from build123d import *

# Parameters (mm, degrees)
SKETCH1_R           = 25
BOSS_EXTRUDE1_DEPTH = 100
SKETCH2_R           = 35
BOSS_EXTRUDE2_DEPTH = 10


with BuildPart() as part:
    # Sketch1 → Boss-Extrude1 (new body)
    with BuildSketch(Plane.XY):
        Circle(SKETCH1_R)
    extrude(amount=BOSS_EXTRUDE1_DEPTH)

    # Sketch2 → Boss-Extrude2 (add)
    with BuildSketch(Plane.XY.offset(100)):
        Circle(SKETCH2_R)
    boss_extrude2 = extrude(amount=BOSS_EXTRUDE2_DEPTH)

    # Mirror1: Boss-Extrude2 across plane
    add(boss_extrude2.mirror(Plane(origin=(0, 0, 50), x_dir=(1, 0, 0), z_dir=(0, 0, -1))))


solid = part.part
Verification items for the finished model (mm, model axes). A direction names the side the tool comes from. Give positions to 0.01 mm unless a question says otherwise; leave off trailing zeros. Loops run counter-clockwise (first coordinate to the right, second up) from the corner with the lowest first, then second, coordinate; pieces in that order, holes last.
1) Sectioned sample at A-A, the plane y = 0. Enter the section's corners in (x, z), then the cut area to 3 significant figures.
2) Sectioned sample at D-D, the plane z = 59.5. Enter the section's corners in (x, y).
3) Draft check along Z on faces 1 (the flat face through (-24, 8, 100)), 2 (the flat face through (0, 0, 110)), 3 (the cylindrical face through (-28, -21, -5)). Enter one of: pulls with the +Z half, pulls with the -Z half, needs draft (parallel to the pull), parting line crosses it, or undercut.
4) Sectioned sample at B-B, the plane x = -30. Enter the section's corners in (y, z), then the cut area to 3 significant figures.
5) Thickness scan on line 1 along Z through (x, y) = (-26, -0.5); line 2 along Y through (x, z) = (1, 64); line 3 along X through (y, z) = (3.5, 88.5). Record the ranges inside material, lowest first.
6) Set-up check for faces 4 (the cylindrical face through (-28, -21, 105)), 5 (the flat face through (-24, 8, 0)): record each of +Z, -Z, +X, -X, +Y, -Y from which the full face is reachable in a straight line by a thin tool's end or side.
7) Depth check by flat-ended pin: pin 1 Ø3 at (x, z) = (-16.5, 3.5) entering from -Y; pin 2 Ø3 at (x, z) = (21, 23) entering from -Y; pin 3 Ø2 at (y, z) = (-5, 82.5) entering from -X. Enter the tip coordinate at first touch or a pass-through.
Answers:
1. outline: (-35, -10) - (35, -10) - (35, 0) - (25, 0) - (25, 100) - (35, 100) - (35, 110) - (-35, 110) - (-35, 100) - (-25, 100) - (-25, 0) - (-35, 0) - close
1. area: 6,400 mm2
2. outline: circle Ø50 at (0, 0)
3. face 1: undercut
3. face 2: pulls with the +Z half
3. face 3: needs draft
4. outline: (-18.03, -10) - (18.03, -10) - (18.03, 0) - (-18.03, 0) - close; (-18.03, 100) - (18.03, 100) - (18.03, 110) - (-18.03, 110) - close
4. area: 721 mm2
5. line 1: z = -10 to 0, 100 to 110
5. line 2: y = -24.98 to 24.98
5. line 3: x = -24.75 to 24.75
6. face 4: +Z, -Z
6. face 5: none
7. pin 1: stops at y = -20
7. pin 2: stops at y = -15.64
7. pin 3: stops at x = -24.68
